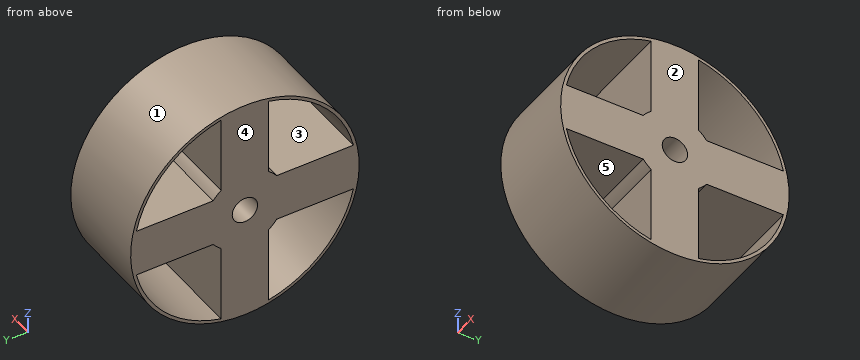
```python
from build123d import *

# Parameters (mm, degrees)
BOSS_EXTRUDE1_DEPTH = 76.2
BOSS_EXTRUDE2_START = -76.2
SKETCH2_R           = 91.44
SKETCH2_R_2         = 88.9
BOSS_EXTRUDE2_DEPTH = 76.2
SKETCH3_R           = 10.16
CUT_EXTRUDE1_DEPTH  = 88.9


with BuildPart() as part:
    # Sketch1 → Boss-Extrude1 (new body)
    with BuildSketch(Plane(origin=(0, 0, 0), x_dir=(0, 0, -1), z_dir=(1, 0, 0))):
        with BuildLine():
            Line((-86.834944003, 19.05), (-25.4, 19.05))
            ThreePointArc((-25.4, 19.05), (-22.450640303, 22.450640303), (-19.05, 25.4))
            Line((-19.05, 25.4), (-19.05, 86.834944003))
            ThreePointArc((-19.05, 86.834944003), (0, 88.9), (19.05, 86.834944003))
            Line((19.05, 86.834944003), (19.05, 25.4))
            ThreePointArc((19.05, 25.4), (22.450640303, 22.450640303), (25.4, 19.05))
            Line((25.4, 19.05), (86.834944003, 19.05))
            ThreePointArc((86.834944003, 19.05), (88.9, 0), (86.834944003, -19.05))
            Line((86.834944003, -19.05), (25.4, -19.05))
            ThreePointArc((25.4, -19.05), (22.450640303, -22.450640303), (19.05, -25.4))
            Line((19.05, -25.4), (19.05, -86.834944003))
            ThreePointArc((19.05, -86.834944003), (0, -88.9), (-19.05, -86.834944003))
            Line((-19.05, -86.834944003), (-19.05, -25.4))
            ThreePointArc((-19.05, -25.4), (-22.450640303, -22.450640303), (-25.4, -19.05))
            Line((-25.4, -19.05), (-86.834944003, -19.05))
            ThreePointArc((-86.834944003, -19.05), (-88.9, 0), (-86.834944003, 19.05))
        make_face()
    extrude(amount=BOSS_EXTRUDE1_DEPTH)

    # Sketch2 → Boss-Extrude2 (add)
    with BuildSketch(Plane(origin=(76.2, 0, 0), x_dir=(0, 0, -1), z_dir=(1, 0, 0)).offset(BOSS_EXTRUDE2_START)):
        Circle(SKETCH2_R)
        Circle(SKETCH2_R_2, mode=Mode.SUBTRACT)
    extrude(amount=BOSS_EXTRUDE2_DEPTH)

    # Sketch3 → Cut-Extrude1 (cut)
    with BuildSketch(Plane(origin=(76.2, 0, 0), x_dir=(0, 0, -1), z_dir=(1, 0, 0))):
        Circle(SKETCH3_R)
    extrude(amount=-CUT_EXTRUDE1_DEPTH, mode=Mode.SUBTRACT)


solid = part.part
```
Here's how the part is built. I have some questions about the finished solid (model axes, mm). Face numbers are marked on the shaded views. A direction names the side the tool comes from. Give positions to 0.01 mm unless a question says otherwise; leave off trailing zeros. Order: outer loops, then holes, each group sorted by start corner. A loop starts at its lowest first (then second) coordinate and runs counter-clockwise, first axis right, second up. Notation, with made-up numbers: M 49,-7 L 91,-7 A18 cw 91,7 Z; hole C -21.5,55.25 d6. An arc over 180 degrees is marked long. Use a Markdown table: item, result. Add a question column.
1. On a 3-axis mill with a long thin cutter (end or side, diameter ignored), from which of +Z, -Z, +X, -X, +Y, -Y can I reach the whole of each face in a straight line? I mean the marked faces 4 and 5. Say none if no direction works.
2. Suppose I cut it at A-A (z = 0). List the corners of the cut face in (x, y) for me, and give its area (3 significant figures).
3. Suppose I cut it at C-C (x = 54.5). List the corners of the cut face in (y, z) for me.
4. I need wall thicknesses on probe 1 along Y at (x, z) = (55, 0); probe 2 along Z at (x, y) = (39.5, -57); probe 3 along Z at (x, y) = (57, 28). Which ranges of each line are inside material? Lowest first, please. Write a range as from..to.
5. Suppose I cut it at D-D (z = 72). List the corners of the cut face in (x, y) for me.
6. For pin 1 Ø18.5 at (x, z) = (46.5, 49) entering from -Y; pin 2 Ø10 at (x, y) = (25.5, 36) entering from +Z; pin 3 Ø10 at (x, z) = (46, 20) entering from -Y, each with a flat end and sliding along its axis, tell me the tip position at first contact or that it passes through.
7. If we mould it in two halves opening along Z, with no side actions, what happens to the marked faces 1, 2 and 3? For each: +Z half, -Z half, draft (parallel to the pull), parting line (faces both ways), or undercut.
Results list:
| question | item | result |
|---|---|---|
| 1 | face 4 | +Z, -Z, -X, +Y, -Y |
| 1 | face 5 | +X, -X |
| 2 | outline | M 0,-91.44 L 76.2,-91.44 L 76.2,-10.16 L 0,-10.16 Z; M 0,10.16 L 76.2,10.16 L 76.2,91.44 L 0,91.44 Z |
| 2 | area | 12,400 mm² |
| 3 | outline | C 0,0 d182.88; hole M -86.83,-19.05 A88.9 ccw -19.05,-86.83 L -19.05,-25.4 A31.75 cw -25.4,-19.05 Z; hole M -86.83,19.05 L -25.4,19.05 A31.75 cw -19.05,25.4 L -19.05,86.83 A88.9 ccw Z; hole C 0,0 d20.32; hole M 19.05,-86.83 A88.9 ccw 86.83,-19.05 L 25.4,-19.05 A31.75 cw 19.05,-25.4 Z; hole M 19.05,25.4 A31.75 cw 25.4,19.05 L 86.83,19.05 A88.9 ccw 19.05,86.83 Z |
| 4 | probe 1 | y = -91.44..-10.16, 10.16..91.44 |
| 4 | probe 2 | z = -71.5..-68.22, -19.05..19.05, 68.22..71.5 |
| 4 | probe 3 | z = -87.05..-84.38, -19.05..19.05, 84.38..87.05 |
| 5 | outline | M 0,-56.37 L 76.2,-56.37 L 76.2,-52.15 L 0,-52.15 Z; M 0,-19.05 L 76.2,-19.05 L 76.2,19.05 L 0,19.05 Z; M 0,52.15 L 76.2,52.15 L 76.2,56.37 L 0,56.37 Z |
| 6 | pin 1 | stops at y = -82.35 |
| 6 | pin 2 | stops at z = 86.02 |
| 6 | pin 3 | stops at y = -90.2 |
| 7 | face 1 | parting line |
| 7 | face 2 | draft |
| 7 | face 3 | undercut |
